The model under review builds one solid part; all positions refer to its coordinate system, in mm. Coordinates: 2 decimals unless noted, no trailing zeros. Order: outer loops, then holes, each group sorted by start corner. A loop starts at its lowest first (then second) coordinate and runs counter-clockwise, first axis right, second up. Notation, with made-up numbers: M 19,85 L 35,85 A14 cw 35,104 Z; hole C 85.25,68.5 d4. An arc over 180 degrees is marked long. Answer in a Markdown table with one row per item.
from build123d import *

# Parameters (mm, degrees)
BOSS_EXTRUDE1_DEPTH      = 60
BOSS_EXTRUDE1_DEPTH_BACK = 20
SKETCH2_R                = 1.7
CUT_EXTRUDE1_DEPTH       = 10
BOSS_EXTRUDE2_START      = 24
BOSS_EXTRUDE2_DEPTH      = 24
SKETCH4_R                = 1.7
CUT_EXTRUDE2_DEPTH       = 24


with BuildPart() as part:
    # Sketch1 → Boss-Extrude1 (new, two sides: drawn at the far end of the back side and taken through both)
    with BuildSketch(Plane(origin=(190.645148, 0, 0), x_dir=(0, 0, -1), z_dir=(1, 0, 0)).offset(-BOSS_EXTRUDE1_DEPTH_BACK)):
        with BuildLine():
            Line((-246.970904961, 208.163538159), (-246.970904961, 205.163538159))
            Line((-246.970904961, 205.163538159), (-246.970904961, 197.163538159))
            Line((-246.970904961, 197.163538159), (-246.970904961, 194.163538159))
            Line((-246.970904961, 194.163538159), (-240.970904961, 194.163538159))
            Line((-240.970904961, 194.163538159), (-240.970904961, 197.163538159))
            Line((-240.970904961, 197.163538159), (-240.970904961, 199.913538158))
            Line((-240.970904961, 199.913538158), (-241.570904961, 199.913538158))
            ThreePointArc((-241.570904961, 199.913538158), (-242.820904961, 201.163538162), (-241.570904955, 202.413538158))
            Line((-241.570904955, 202.413538158), (-240.970904961, 202.413538158))
            Line((-240.970904961, 202.413538158), (-240.970904961, 205.163538159))
            Line((-240.970904961, 205.163538159), (-240.970904961, 208.163538159))
            Line((-240.970904961, 208.163538159), (-246.970904961, 208.163538159))
        make_face()
    extrude(amount=BOSS_EXTRUDE1_DEPTH + BOSS_EXTRUDE1_DEPTH_BACK)

    # Sketch2 → Cut-Extrude1 (cut)
    with BuildSketch(Plane.XY.offset(246.970904961)):
        with Locations((246.645148, 197.663538159)):
            Circle(SKETCH2_R)
        with Locations((198.645148, 197.663538159)):
            Circle(SKETCH2_R)
        with Locations((174.645148, 197.663538159)):
            Circle(SKETCH2_R)
        with Locations((222.645148, 197.663538159)):
            Circle(SKETCH2_R)
        with Locations((174.645148, 204.663538159)):
            Circle(SKETCH2_R)
        with Locations((198.645148, 204.663538159)):
            Circle(SKETCH2_R)
        with Locations((222.645148, 204.663538159)):
            Circle(SKETCH2_R)
        with Locations((246.645148, 204.663538159)):
            Circle(SKETCH2_R)
    extrude(amount=-CUT_EXTRUDE1_DEPTH, mode=Mode.SUBTRACT)

    # Sketch3 → Boss-Extrude2 (add)
    with BuildSketch(Plane.ZY.offset(-170.645148).offset(BOSS_EXTRUDE2_START)):
        with BuildLine():
            Line((246.970904961, 208.163538159), (240.970904961, 208.163538159))
            Line((240.970904961, 208.163538159), (240.970904961, 202.413538158))
            Line((240.970904961, 202.413538158), (241.570904955, 202.413538158))
            ThreePointArc((241.570904955, 202.413538158), (242.820904961, 201.163538162), (241.570904961, 199.913538158))
            Line((241.570904961, 199.913538158), (240.970904961, 199.913538158))
            Line((240.970904961, 199.913538158), (240.970904961, 194.163538159))
            Line((240.970904961, 194.163538159), (246.970904961, 194.163538159))
            Line((246.970904961, 194.163538159), (246.970904961, 208.163538159))
        make_face()
    extrude(amount=-BOSS_EXTRUDE2_DEPTH)

    # Sketch4 → Cut-Extrude2 (cut)
    with BuildSketch(Plane.XY.offset(246.970904961)):
        with Locations((150.645148, 197.663538159)):
            Circle(SKETCH4_R)
        with Locations((150.645148, 204.663538159)):
            Circle(SKETCH4_R)
    extrude(amount=-CUT_EXTRUDE2_DEPTH, mode=Mode.SUBTRACT)


solid = part.part
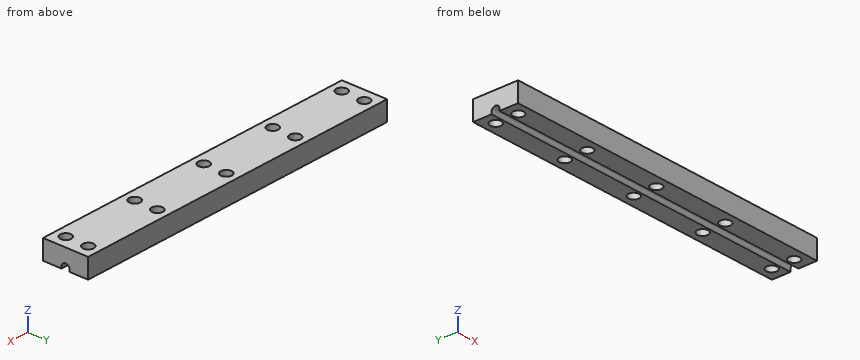
(1) Take a section at C-C (y = 201.5). Write out the cut boundary in (x, z).
Report:
| item | result |
|---|---|
| outline | M 146.65,242.77 L 250.65,242.77 L 250.65,246.97 L 146.65,246.97 Z |
(2) Take a section at B-B (x = 161). Write out the cut boundary in (y, z).
Report:
| item | result |
|---|---|
| outline | M 194.16,240.97 L 199.91,240.97 L 199.91,241.57 A1.25 cw 202.41,241.57 L 202.41,240.97 L 208.16,240.97 L 208.16,246.97 L 194.16,246.97 Z |
(3) To check wall thickness, follow line 1 (X direction, y = 204.75, z = 244.4); line 2 (X direction, y = 203.5, z = 243.4); line 3 (Y direction, x = 172, z = 241.35). State the ranges of each line that lie inside material, in increasing order. Write a range as [from, to].
Report:
| item | result |
|---|---|
| line 1 | [146.65, 148.95], [152.34, 172.95], [176.34, 196.95], [200.34, 220.95], [224.34, 244.95], [248.34, 250.65] |
| line 2 | [146.65, 149.41], [151.88, 173.41], [175.88, 197.41], [199.88, 221.41], [223.88, 245.41], [247.88, 250.65] |
| line 3 | [194.16, 199.91], [202.41, 208.16] |
(4) Insertion check: P1, Ø4, axis at x = 246.65, y = 197.66, coming from the +Z side. The pin has a flat end and moves straight along its axis. Give the tip position at first contact, or say it passes through.
Report:
| item | result |
|---|---|
| P1 | z = 246.97 |
(5) Take a section at A-A (z = 245.7). State how many separate pieces and enclosed holes the cut face has, then the cut area to 3 significant figures.
Report:
| item | result |
|---|---|
| separate pieces | 1 |
| enclosed holes | 10 |
| area | 1,370 mm^2 |
